Drawing for the job (mm, zero at the part's lowest x, y, z). Round coordinates to 2 decimals unless told otherwise and drop trailing zeros. Write each loop counter-clockwise with the first axis right and the second up, starting at its lowest first coordinate (ties: lowest second). Pieces come first, ordered by that corner, then holes.
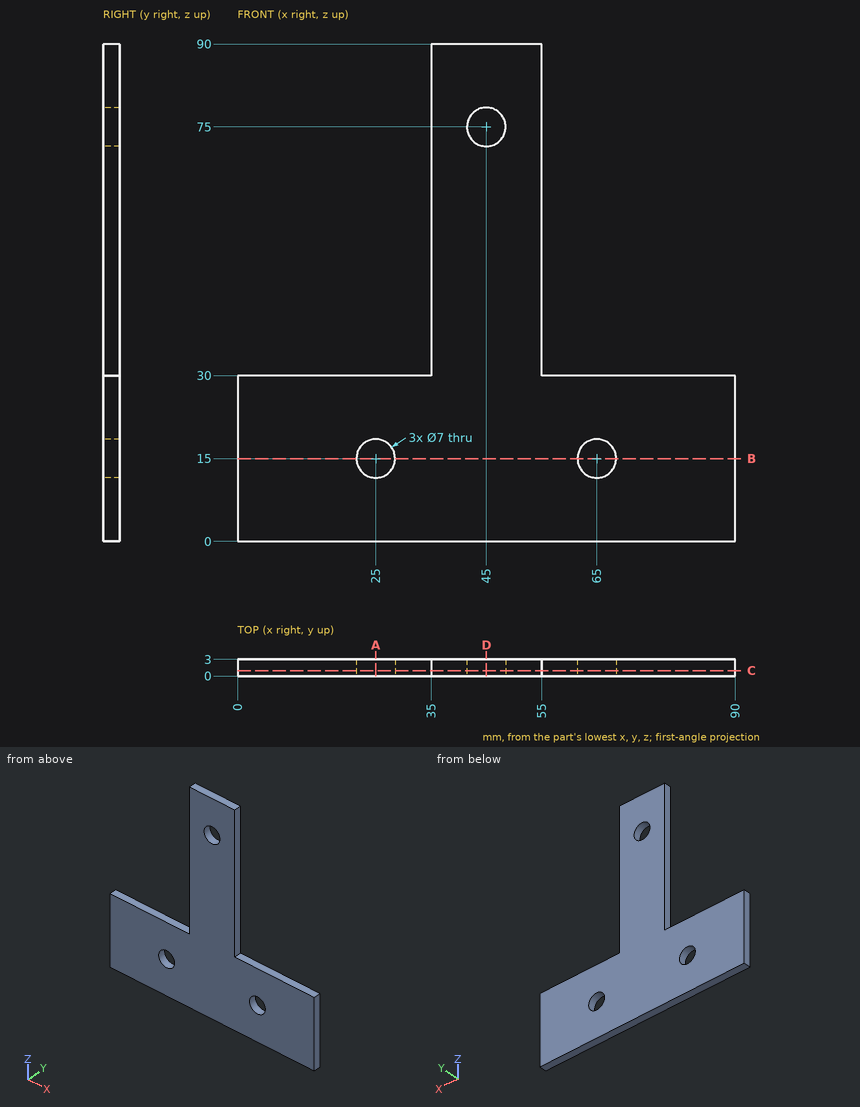
1) Cut at C-C on y = 0.95. List the corners of the cut face in (x, z).
2) Flat gauge pins, fed straight in: pin 1 Ø1 at (x, y) = (47, 2) entering from -Z; pin 2 Ø1 at (y, z) = (2, 36) entering from -X; pin 3 Ø1.5 at (y, z) = (2, 64) entering from +X; pin 4 Ø1.5 at (x, z) = (56.5, 52) entering from +Y. Where does each tip first touch, or does it go through?
3) Cut at A-A on x = 25. List the corners of the cut face in (y, z).
4) Cut at B-B on z = 15. List the corners of the cut face in (x, y).
5) Cut at D-D on x = 45. List the corners of the cut face in (y, z), and give its area (3 significant figures).
6) Wall check: probe 1 along X at (y, z) = (1.55, 15); probe 2 along X at (y, z) = (1.6, 75); probe 3 along Z at (x, y) = (65, 2.3). Give the ranges that are in metal, low to high.
Result sheet:
1. outline: (0, 0) - (90, 0) - (90, 30) - (55, 30) - (55, 90) - (35, 90) - (35, 30) - (0, 30) - close; hole circle Ø7 at (25, 15); hole circle Ø7 at (45, 75); hole circle Ø7 at (65, 15)
2. pin 1: stops at z = 0
2. pin 2: stops at x = 35
2. pin 3: stops at x = 55
2. pin 4: passes through
3. outline: (0, 0) - (3, 0) - (3, 11.5) - (0, 11.5) - close; (0, 18.5) - (3, 18.5) - (3, 30) - (0, 30) - close
4. outline: (0, 0) - (21.5, 0) - (21.5, 3) - (0, 3) - close; (28.5, 0) - (61.5, 0) - (61.5, 3) - (28.5, 3) - close; (68.5, 0) - (90, 0) - (90, 3) - (68.5, 3) - close
5. outline: (0, 0) - (3, 0) - (3, 71.5) - (0, 71.5) - close; (0, 78.5) - (3, 78.5) - (3, 90) - (0, 90) - close
5. area: 249 mm2
6. probe 1: x = 0 to 21.5, 28.5 to 61.5, 68.5 to 90
6. probe 2: x = 35 to 41.5, 48.5 to 55
6. probe 3: z = 0 to 11.5, 18.5 to 30
